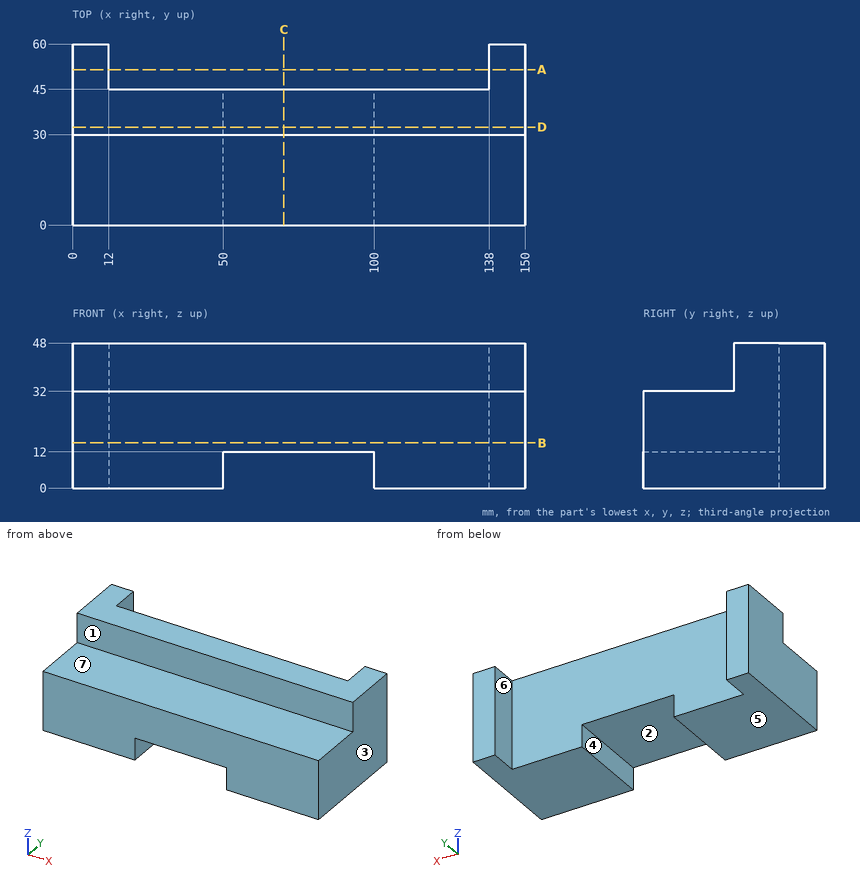
Study the drawing (mm; zero at the part's minimum x, y, z) and answer. A direction names the side the tool comes from. Give positions to 0.01 mm unless a question says otherwise; leave off trailing zeros. Write each loop counter-clockwise with the first axis right and the second up, starting at its lowest first coordinate (ties: lowest second). Pieces come first, ordered by that corner, then holes. Notation, with made-up numbers: (3.5, -15) -> (48.5, -15) arc R20 cw to (48.5, 22) -> close; hole circle Ø2 at (-14.5, 18.5). An arc over 180 degrees is marked (long way). Write item = value, one per line. Start each with the question number.
1) Which of the six approach directions +Z, -Z, +X, -X, +Y, -Y give full straight-line access (tool end or side, diameter ignored) to the marked faces 4, 5, 6 and 7?
2) The part is cut by section B-B, the plane z = 15. Determine the outline of the cut face in (x, y), and give its area (3 significant figures).
3) Straight lines are drawn through the part: line 1 along X through (y, z) = (18.5, 2); line 2 along X through (y, z) = (56.5, 34.5); line 3 along Y through (x, z) = (88, 44.5). For each, find the intervals that lie inside material, in ascending order.
4) The part is cut by section A-A, the plane y = 51.5. Determine the outline of the cut face in (x, z), and give its area (3 significant figures).
5) The part is cut by section C-C, the plane x = 70. Determine the outline of the cut face in (y, z), and give its area (3 significant figures).
6) The part is cut by section D-D, the plane y = 32.5. Determine the outline of the cut face in (x, z).
7) Determine the mould class of the marked faces 1, 2 and 3 for opening direction X: +X half, -X half, draft (parallel to the pull), parting line (faces both ways), or undercut.
8) Each of these flat-tipped pins is pushed along its axis until it touches: pin 1 (4 mm diameter, centred on x = 105.5, z = 38, fed in from +Y); pin 2 (8 mm diameter, centred on x = 79.5, y = 48, fed in from -Z); pin 3 (24 mm diameter, centred on x = 69, y = 12.5, fed in from +Z). Where does it stop, or does it pass through?
Solutions:
q1.face_4 = -Z, +Y, -Y
q1.face_5 = -Z, +X, -X, +Y, -Y
q1.face_6 = +Z, -Z, +Y
q1.face_7 = +Z, +X, -X, -Y
q2.outline = (0, 0) -> (150, 0) -> (150, 60) -> (138, 60) -> (138, 45) -> (12, 45) -> (12, 60) -> (0, 60) -> close
q2.area = 7,110 mm²
q3.line_1 = 0 to 50, 100 to 150
q3.line_2 = 0 to 12, 138 to 150
q3.line_3 = 30 to 45
q4.outline = (0, 0) -> (12, 0) -> (12, 48) -> (0, 48) -> close; (138, 0) -> (150, 0) -> (150, 48) -> (138, 48) -> close
q4.area = 1,150 mm²
q5.outline = (0, 12) -> (45, 12) -> (45, 48) -> (30, 48) -> (30, 32) -> (0, 32) -> close
q5.area = 1,140 mm²
q6.outline = (0, 0) -> (50, 0) -> (50, 12) -> (100, 12) -> (100, 0) -> (150, 0) -> (150, 48) -> (0, 48) -> close
q7.face_1 = draft
q7.face_2 = undercut
q7.face_3 = +X half
q8.pin_1 = 45
q8.pin_2 = 12
q8.pin_3 = 32
